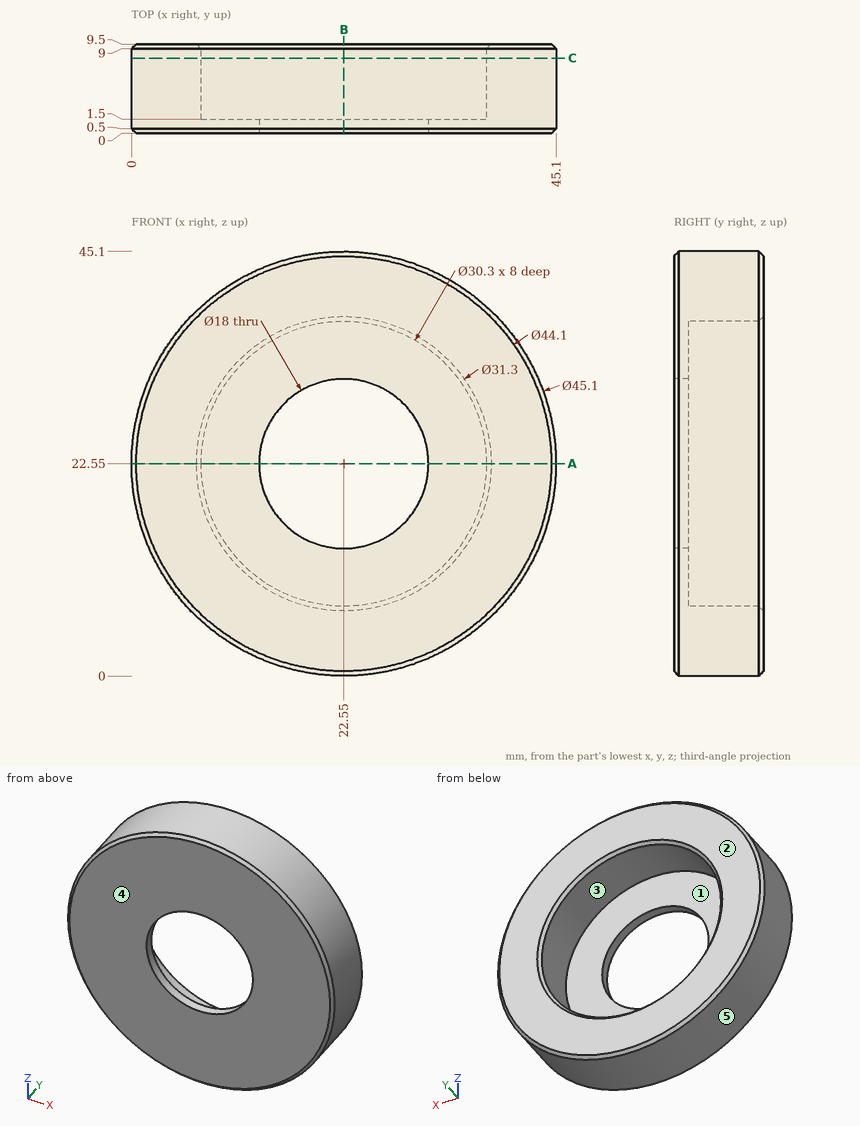
Study the drawing (mm; zero at the part's minimum x, y, z) and answer. A direction names the side the tool comes from. Round coordinates to 2 decimals unless told otherwise and drop trailing zeros. Order: outer loops, then holes, each group sorted by start corner. A loop starts at its lowest first (then second) coordinate and runs counter-clockwise, first axis right, second up. Notation, with made-up numbers: (89.5, 81) -> (94.5, 81) arc R32 cw to (94.5, 109) -> close; hole circle Ø4 at (37, 40). An arc over 180 degrees is marked (long way). Write each question's results on one line, items separated by ' | '. Start each with the question number.
Q1. The mould has two halves that part along Z. Classify the marked faces 3, 4 and 5: pulls with the +Z half, pulls with the -Z half, needs draft (parallel to the pull), parting line crosses it, or undercut.
Q2. Find section C-C (y = 8). Determine the outline of the cut face in (x, z), then the cut area to 3 significant figures.
Q3. Find section B-B (x = 22.55). Determine the outline of the cut face in (y, z).
Q4. Which of the six approach directions +Z, -Z, +X, -X, +Y, -Y give full straight-line access (tool end or side, diameter ignored) to the marked faces 1 and 2?
Q5. Straight lines are drawn through the part: probe 1 along Z at (x, y) = (22.55, 0.6); probe 2 along Z at (x, y) = (22.55, 4.5); probe 3 along Y at (x, z) = (20.5, 35). For each, find the intervals that lie inside material, in ascending order. Write a range as from..to.
Q6. Find section A-A (z = 22.55). Determine the outline of the cut face in (x, y).
Q7. Each of these flat-tipped pins is pushed along its axis until it touches: pin 1 (1.5 mm diameter, centred on x = 16, y = 8, fed in from +Z); pin 2 (2 mm diameter, centred on x = 38.5, y = 3.5, fed in from -Z); pin 3 (5 mm diameter, centred on x = 29, z = 13, fed in from +Y). Where does it stop, or does it pass through?
Worked answers:
1) face 3: undercut | face 4: needs draft | face 5: parting line crosses it
2) outline: circle Ø45.1 at (22.55, 22.55); hole circle Ø30.3 at (22.55, 22.55) | area: 876 mm2
3) outline: (0, 0.5) -> (0.5, 0) -> (9, 0) -> (9.5, 0.5) -> (9.5, 6.9) -> (9, 7.4) -> (1.5, 7.4) -> (1.5, 13.55) -> (0, 13.55) -> close; (0, 31.55) -> (1.5, 31.55) -> (1.5, 37.7) -> (9, 37.7) -> (9.5, 38.2) -> (9.5, 44.6) -> (9, 45.1) -> (0.5, 45.1) -> (0, 44.6) -> close
4) face 1: +Y | face 2: +Z, -Z, +X, -X, +Y
5) probe 1: z = 0..13.55, 31.55..45.1 | probe 2: z = 0..7.4, 37.7..45.1 | probe 3: y = 0..1.5
6) outline: (0, 0.5) -> (0.5, 0) -> (13.55, 0) -> (13.55, 1.5) -> (7.4, 1.5) -> (7.4, 9) -> (6.9, 9.5) -> (0.5, 9.5) -> (0, 9) -> close; (31.55, 0) -> (44.6, 0) -> (45.1, 0.5) -> (45.1, 9) -> (44.6, 9.5) -> (38.2, 9.5) -> (37.7, 9) -> (37.7, 1.5) -> (31.55, 1.5) -> close
7) pin 1: stops at z = 44.34 | pin 2: stops at z = 5.67 | pin 3: stops at y = 1.5
